```python
from build123d import *

# Parameters (mm, degrees)
F1_DEPTH  = 27
F2_DEPTH  = 8
F4_DEPTH  = 22
F6_R      = 2
F8_DEPTH  = 20
F9_DEPTH  = 12.5
F5_R      = 2.5
F10_DEPTH = 2.4607981127
F11_DEPTH = 12.5


with BuildPart() as f1:
    # F0 (on Front) → F1 (new body)
    with BuildSketch(Plane.XZ):
        Polygon((-0.7496952344, -6.6809873255), (0.8741063205, -6.6809873255), (0.9227698261, -6.0829417354), (0, -5.9686545786), (-0.1947072298, -5.7400796882), (-0.1947072298, -5.5496009013), (-0.1947072298, -5.0035609814), (0.1608536688, -5.0035609814), (0.8973725199, -4.86387623), (1.0449768405, -4.7641876783), (1.0008919092, -2.5655001409), (0.9438757817, -2.5243218008), (-0.1411063758, -2.4221134883), (-0.2590392278, -2.3199048873), (-0.3769720528, -2.1705233078), (-0.3769720528, -1.9110710604), (-0.266901421, -1.7774139032), (-0.0703466601, -1.5729969897), (0.1891055828, -1.3843043544), (0.9716137966, -1.1052864284), (0.9130675168, 1.8146449861), (-1.3546038697, 1.7419207949), (-1.3418151463, 0.7710934816), (-1.1574519325, 0.707130723), (-0.1783869789, 0.5052616682), (0, 0.2579721058), (0.0436689517, 0.1116170257), (0.0436689517, -0.0700651218), (0, -0.439608231), (-0.1037999714, -0.6445581556), (-1.2615459958, -0.9208470772), (-1.2615459958, -3.1862834304), (0, -3.5216339192), (0, -4.1217343841), (-1.2262458836, -4.457084873), (-1.2262458836, -6.5044873415), align=None)
    extrude(amount=-F1_DEPTH)

    # F0 (on Front) → F2 (join)
    with BuildSketch(Plane.XZ):
        Polygon((-0.7496952344, -6.6809873255), (0.8741063205, -6.6809873255), (0.9227698261, -6.0829417354), (0, -5.9686545786), (-0.1947072298, -5.7400796882), (-0.1947072298, -5.5496009013), (-0.1947072298, -5.0035609814), (0.1608536688, -5.0035609814), (0.8973725199, -4.86387623), (1.0449768405, -4.7641876783), (1.0008919092, -2.5655001409), (0.9438757817, -2.5243218008), (-0.1411063758, -2.4221134883), (-0.2590392278, -2.3199048873), (-0.3769720528, -2.1705233078), (-0.3769720528, -1.9110710604), (-0.266901421, -1.7774139032), (-0.0703466601, -1.5729969897), (0.1891055828, -1.3843043544), (0.9716137966, -1.1052864284), (0.9130675168, 1.8146449861), (-1.3546038697, 1.7419207949), (-1.3418151463, 0.7710934816), (-1.1574519325, 0.707130723), (-0.1783869789, 0.5052616682), (0, 0.2579721058), (0.0436689517, 0.1116170257), (0.0436689517, -0.0700651218), (0, -0.439608231), (-0.1037999714, -0.6445581556), (-1.2615459958, -0.9208470772), (-1.2615459958, -3.1862834304), (0, -3.5216339192), (0, -4.1217343841), (-1.2262458836, -4.457084873), (-1.2262458836, -6.5044873415), align=None)
        Polygon((0.9227698261, -6.0829417354), (0.8741063205, -6.6809873255), (-0.7496952344, -6.6809873255), (-1.2262458836, -6.5044873415), (-1.2262458836, -4.457084873), (0, -4.1217343841), (0, -3.5216339192), (-1.2615459958, -3.1862834304), (-1.2615459958, -0.9208470772), (-0.1037999714, -0.6445581556), (0, -0.439608231), (0.0436689517, -0.0700651218), (0.0436689517, 0.1116170257), (0, 0.2579721058), (-0.1783869789, 0.5052616682), (-1.1574519325, 0.707130723), (-1.3418151463, 0.7710934816), (-1.2262458836, -8.0020884052), (1.1092817108, -7.9713224635), (1.0449768405, -4.7641876783), (0.8973725199, -4.86387623), (0.1608536688, -5.0035609814), (-0.1947072298, -5.0035609814), (-0.1947072298, -5.5496009013), (-0.1947072298, -5.7400796882), (0, -5.9686545786), align=None)
        Polygon((0.9438757817, -2.5243218008), (1.0008919092, -2.5655001409), (0.9716137966, -1.1052864284), (0.1891055828, -1.3843043544), (-0.0703466601, -1.5729969897), (-0.266901421, -1.7774139032), (-0.3769720528, -1.9110710604), (-0.3769720528, -2.1705233078), (-0.2590392278, -2.3199048873), (-0.1411063758, -2.4221134883), align=None)
    extrude(amount=F2_DEPTH)

    # F3 (on face) → F4 (join)
    with BuildSketch(Plane.XZ.offset(8)):
        Polygon((0.7385039935, 6.1391890049), (-1.3546038697, 6.1391890049), (-1.3316788356, 1.7426560004), (0.8252700079, 1.8118293212), align=None)
        Polygon((0.8252700079, 1.8118293212), (-1.3316788356, 1.7426560004), (-1.3166525213, -1.1390708706), (-1.2262458836, -8.0020884052), (1.0214509446, -7.9724794596), align=None)
        Polygon((-1.2262458836, -8.0020884052), (-1.3166525213, -1.1390708706), (-1.2591139525, -12.1737421996), (1.1047383155, -12.1263456218), (1.0214509446, -7.9724794596), align=None)
    extrude(amount=F4_DEPTH)

    # F6
    f6_edges = [f1.edges().sort_by_distance(p)[0] for p in [
        (-0.30805, -30, 6.139189),
        (-0.077188, -30, -12.150044),
        (-0.30805, -8, 6.139189),
        (-0.077188, -8, -12.150044),
    ]]
    fillet(f6_edges, radius=F6_R)

    # F7 (on Right) → F8 (cut, symmetric)
    with BuildSketch(Plane.YZ):
        Polygon((6.4942785373, -3.7844735536), (4.42, -2.3853550139), (0, -5.5966729877), (-11.7603398875, -14.1410600597), (31.9972857833, -14.0815703198), (31.4160363876, 5.4046616789), (20.8858734821, 5.4046616789), (28.2785118313, 0.4182641504), (22.4941027949, -3.7843550139), (20.42, -2.3853550139), (18.4942785373, -3.7844735536), (16.42, -2.3853550139), (14.4942785373, -3.7844735536), (12.42, -2.3853550139), (10.4942785373, -3.7844735536), (8.42, -2.3853550139), align=None)
    extrude(amount=F8_DEPTH, both=True, mode=Mode.SUBTRACT)

    # F7 (on Right) → F9 (cut, symmetric)
    with BuildSketch(Plane.YZ):
        Polygon((6.4942785373, -3.7844735536), (4.42, -2.3853550139), (0, -5.5966729877), (-11.7603398875, -14.1410600597), (31.9972857833, -14.0815703198), (31.4160363876, 5.4046616789), (20.8858734821, 5.4046616789), (28.2785118313, 0.4182641504), (22.4941027949, -3.7843550139), (20.42, -2.3853550139), (18.4942785373, -3.7844735536), (16.42, -2.3853550139), (14.4942785373, -3.7844735536), (12.42, -2.3853550139), (10.4942785373, -3.7844735536), (8.42, -2.3853550139), align=None)
    extrude(amount=F9_DEPTH, both=True, mode=Mode.SUBTRACT)

    # F5 (on face) → F10 (cut, through all)
    with BuildSketch(Plane(origin=(0.8612519677, 0, 0.0172685901), x_dir=(0, 1, 0), z_dir=(0.999799048, 0, 0.0200465376))):
        with Locations((-25.5, 1.6231508744)):
            Circle(F5_R)
    extrude(amount=-F10_DEPTH, mode=Mode.SUBTRACT)

    # F7 (on Right) → F11 (cut, symmetric)
    with BuildSketch(Plane.YZ):
        Polygon((6.4942785373, -3.7844735536), (4.42, -2.3853550139), (0, -5.5966729877), (-11.7603398875, -14.1410600597), (31.9972857833, -14.0815703198), (31.4160363876, 5.4046616789), (20.8858734821, 5.4046616789), (28.2785118313, 0.4182641504), (22.4941027949, -3.7843550139), (20.42, -2.3853550139), (18.4942785373, -3.7844735536), (16.42, -2.3853550139), (14.4942785373, -3.7844735536), (12.42, -2.3853550139), (10.4942785373, -3.7844735536), (8.42, -2.3853550139), align=None)
    extrude(amount=F11_DEPTH, both=True, mode=Mode.SUBTRACT)


solid = f1.part
```
For this review, take the finished solid that the model builds, in its own axes (mm). A direction names the side the tool comes from. Round coordinates to 2 decimals unless told otherwise and drop trailing zeros. Write each loop counter-clockwise with the first axis right and the second up, starting at its lowest first coordinate (ties: lowest second). Pieces come first, ordered by that corner, then holes. Notation, with made-up numbers: (73.25, -8.5) -> (93.25, -8.5) arc R32 ccw to (93.25, 29.5) -> close; hole circle Ø6 at (-2, -31.75). An arc over 180 degrees is marked (long way). Use one line per item in the form item = value.
1) Mouldability with a two-part tool opening along Y and no side actions: class faces 4 (the flat face through (-0.675, 13.311, 0.608)), 5 (the flat face through (-0.102, 7.471, -3.075)), 6 (the flat face through (0, -8, -9)) as +Y half, -Y half, draft (parallel to the pull), parting line (faces both ways), or undercut.
Found:
face_4 = draft
face_5 = undercut
face_6 = +Y half
2) Take a section at C-C, the plane z = -6.5. Write out the cut boundary in (x, y).
Found:
outline = (-1.29, -30) -> (0.99, -30) -> (0.99, -8) -> (1.08, -8) -> (1.08, -1.24) -> (-1.25, -1.24) -> (-1.25, -8) -> (-1.29, -8) -> close
3) Take a section at A-A, the plane y = -24.5. Write out the cut boundary in (x, z).
Found:
outline = (-1.35, 6.14) -> (-1.34, 3.89) -> (0.78, 3.93) -> (0.74, 6.14) -> close; (-1.32, -0.69) -> (-1.26, -12.17) -> (1.1, -12.13) -> (0.87, -0.65) -> close
4) To check wall thickness, follow L1, parallel to Y at x = -0.3, z = -3; L2, parallel to Y at x = -0.1, z = -9; L3, parallel to X at y = -25.5, z = -8.75. State the ranges of each line that lie inside material, in increasing order. Write a range as from..to.
Found:
L1 = -30..3.57, 5.33..7.57, 9.33..11.57, 13.33..15.57, 17.33..19.57, 21.33..23.57
L2 = -30..-8
L3 = -1.28..1.04
5) Take a section at B-B, the plane y = -6. Write out the cut boundary in (x, z).
Found:
outline = (-1.35, 1.74) -> (-1.23, -8) -> (1.11, -7.97) -> (0.91, 1.81) -> close
6) Take a section at D-D, the plane z = -9. Write out the cut boundary in (x, y).
Found:
outline = (-1.28, -30) -> (1.04, -30) -> (1.04, -8) -> (-1.28, -8) -> close
7) Clearance check with flat-ended pins moving along their axes: pin 1 (0.7 mm diameter, centred on x = -0.5, z = 3.5, fed in from +Y); pin 2 (3 mm diameter, centred on y = -16.5, z = 1.5, fed in from +X); pin 3 (1.1 mm diameter, centred on x = -0.5, z = -2.5, fed in from +Y). State where each tip first meets the part, or that it passes through.
Found:
pin_1 = -8
pin_2 = 0.86
pin_3 = 25.02
8) Tool access review of faces 1 (the flat face through (-0.78, 18.451, -3.314)), 2 (the flat face through (0.409, 2.154, -2.474)), 3 (the flat face through (-0.102, 21.472, -3.095)): name each direction out of +Z, -Z, +X, -X, +Y, -Y from which nothing blocks a thin tool from reaching the whole face with its end or side.
Found:
face_1 = -Z, -X, +Y
face_2 = +X, +Y
face_3 = -Z, +X, -X
